Input: part model. Units: mm. Frame: model coordinates. A direction names the side the tool comes from. Give positions to 0.01 mm unless a question says otherwise; leave off trailing zeros. Loops run counter-clockwise (first coordinate to the right, second up) from the corner with the lowest first, then second, coordinate; pieces in that order, holes last. Notation, with made-up numbers: (-27, 37) -> (-18, 37) arc R5 ccw to (-18, 41) -> close; hole circle Ø8 at (-29, 60.25). An arc over 180 degrees is marked (long way). Answer as a JSON object with one key per item and string values. Group by question number.
```python
from build123d import *

# Parameters (mm, degrees)
SKETCH1_R                   = 11
FLANGE_DEPTH                = 2
SKETCH2_R                   = 5
COLLAR_DEPTH                = 10
SKETCH3_R                   = 3
CUT_EXTRUDE1_DEPTH          = 20.646882704
SET_SCREW_TAP_1_D           = 2.5
SET_SCREW_TAP_1_DEPTH       = 5
SET_SCREW_TAP_1_CSINK_D     = 2.55
SET_SCREW_TAP_1_CSINK_ANGLE = 90
SET_SCREW_TAP_2_D           = 2.5
SET_SCREW_TAP_2_DEPTH       = 8.001
SET_SCREW_TAP_2_CSINK_D     = 2.55
SET_SCREW_TAP_2_CSINK_ANGLE = 90
FLANGE_HOLES_AT_2_COUNT     = 2
FLANGE_HOLES_AT_2_PITCH     = 8
FLANGE_HOLES_AT_3_COUNT     = 2
FLANGE_HOLES_AT_3_PITCH     = 8
FLANGE_HOLES_AT_4_COUNT     = 2
FLANGE_HOLES_AT_4_PITCH     = 8
FLANGE_HOLES_AT_5_COUNT     = 2
FLANGE_HOLES_AT_5_PITCH     = 8
BODY_CHAMFERS_SIZE          = 0.2


with BuildPart() as part:
    # Sketch1 → Flange (new body)
    with BuildSketch(Plane(origin=(0, 0, 0), x_dir=(1, 0, 0), z_dir=(0, 1, 0))):
        with Locations(Location((0, 0, 0), (0, 0, 270))):
            Circle(SKETCH1_R)
    extrude(amount=FLANGE_DEPTH)

    # Sketch2 → Collar (add)
    with BuildSketch(Plane(origin=(0, 2, 0), x_dir=(1, 0, 0), z_dir=(0, 1, 0))):
        with Locations(Location((0, 0, 0), (0, 0, 270))):
            Circle(SKETCH2_R)
    extrude(amount=COLLAR_DEPTH)

    # Sketch3 → Cut-Extrude1 (cut, through all)
    with BuildSketch(Plane(origin=(0, 12, 0), x_dir=(1, 0, 0), z_dir=(0, 1, 0))):
        with Locations(Location((0, 0, 0), (0, 0, 270))):
            Circle(SKETCH3_R)
    extrude(amount=-CUT_EXTRUDE1_DEPTH, mode=Mode.SUBTRACT)

    # Set Screw Tap 1
    with Locations(Plane(origin=(5, 8.85, 0), x_dir=(0, 0, 1), z_dir=(1, 0, 0))):
        with Locations((0, 0)):
            CounterSinkHole(SET_SCREW_TAP_1_D / 2, SET_SCREW_TAP_1_CSINK_D / 2, depth=SET_SCREW_TAP_1_DEPTH, counter_sink_angle=SET_SCREW_TAP_1_CSINK_ANGLE)

    # Set Screw Tap 2
    with Locations(Plane(origin=(-5, 8.85, 0), x_dir=(0, 0, -1), z_dir=(-1, 0, 0))):
        with Locations((0, 0)):
            CounterSinkHole(SET_SCREW_TAP_2_D / 2, SET_SCREW_TAP_2_CSINK_D / 2, depth=SET_SCREW_TAP_2_DEPTH, counter_sink_angle=SET_SCREW_TAP_2_CSINK_ANGLE)

    # Sketch11 → Flange Holes (revolve, cut)
    with BuildSketch(Plane(origin=(0, 2, 0), x_dir=(0, 0, 1), z_dir=(1, 0, 0))):
        Polygon((0, 0), (0, 2), (1.625, 2), (1.5, 1.875), (1.5, 0.125), (1.625, 0), align=None)
    flange_holes = revolve(axis=Axis((0, 8.35, 0), (0, -1, 0)), mode=Mode.SUBTRACT)

    # Flange Holes at 2: Flange Holes ×2
    with Locations(*[Vector(-0.7071067811865476, 0, -0.7071067811865476) * (i * FLANGE_HOLES_AT_2_PITCH) for i in range(1, FLANGE_HOLES_AT_2_COUNT)]):
        add(flange_holes, mode=Mode.SUBTRACT)

    # Flange Holes at 3: Flange Holes ×2
    with Locations(*[Vector(-0.7071067811865476, 0, 0.7071067811865476) * (i * FLANGE_HOLES_AT_3_PITCH) for i in range(1, FLANGE_HOLES_AT_3_COUNT)]):
        add(flange_holes, mode=Mode.SUBTRACT)

    # Flange Holes at 4: Flange Holes ×2
    with Locations(*[Vector(0.7071067811865476, 0, 0.7071067811865476) * (i * FLANGE_HOLES_AT_4_PITCH) for i in range(1, FLANGE_HOLES_AT_4_COUNT)]):
        add(flange_holes, mode=Mode.SUBTRACT)

    # Flange Holes at 5: Flange Holes ×2
    with Locations(*[Vector(0.7071067811865476, 0, -0.7071067811865476) * (i * FLANGE_HOLES_AT_5_PITCH) for i in range(1, FLANGE_HOLES_AT_5_COUNT)]):
        add(flange_holes, mode=Mode.SUBTRACT)

    # Body Chamfers
    body_chamfers_edges = [part.edges().sort_by_distance(p)[0] for p in [
        (0, 0, -3),
        (0, 12, -3),
        (0, 0, -11),
        (0, 2, -11),
        (0, 2, -5),
        (0, 12, -5),
    ]]
    chamfer(body_chamfers_edges, length=BODY_CHAMFERS_SIZE)


solid = part.part
```
Q1. Set-up query: faces 5 (the face through (4.64, 1.01, -6.76)), 6 (the face through (3, 2, 5)). Return all of +Z, -Z, +X, -X, +Y, -Y with unobstructed straight access to the full face (end or side cutting, diameter ignored); none if empty.
Q2. Section D-D on y = 5.5. Return the cut outline in (x, z), then the cut area to 3 significant figures.
Q3. Section A-A on x = 0. Return the cut outline in (y, z).
Q4. Ray query, probe 1 along Y at (x, z) = (3.45, 0); probe 2 along Y at (x, z) = (-1.5, 5.75); probe 3 along X at (y, z) = (10, -1.25). Return the intervals inside material, ascending.
Q5. Section C-C on y = 9.5. Return the cut outline in (x, z).
Q6. Section B-B on z = 0. State how many separate pieces and enclosed holes the cut face has, then the cut area to 3 significant figures.
Q7. Pin query (flat end, axial travel): pin 1 Ø1.5 at (x, z) = (-7, 1.5) entering from -Y; pin 2 Ø3 at (y, z) = (10, -2.5) entering from -X; pin 3 Ø6 at (y, z) = (10.5, 7.5) entering from -X; pin 4 Ø2 at (x, y) = (-3, 4.5) entering from -Z. Return the tip coordinate at first contact, or that it passes through.
Q8. Pull-direction query (X, two-part tool) for faces 1 (the face through (4.17, 1.01, 5.46)), 2 (the face through (3.835, 9.959, -0.577)), 3 (the face through (-4.436, 6.933, 2.307)), 4 (the face through (-4.744, 1.012, -6.847)); classes: +X half, -X half, draft (parallel to the pull), parting line (faces both ways), or undercut.
Numbers:
{
 "1": {"face 5": "+Y, -Y", "face 6": "+Y"},
 "2": {"outline": "circle Ø10 at (0, 0); hole circle Ø6 at (0, 0)", "area": "50.3 mm²"},
 "3": {"outline": "(0, -10.8) -> (0.2, -11) -> (1.8, -11) -> (2, -10.8) -> (2, -5.2) -> (2.2, -5) -> (11.8, -5) -> (12, -4.8) -> (12, -3.2) -> (11.8, -3) -> (0.2, -3) -> (0, -3.2) -> close; (0, 3.2) -> (0.2, 3) -> (11.8, 3) -> (12, 3.2) -> (12, 4.8) -> (11.8, 5) -> (2.2, 5) -> (2, 5.2) -> (2, 10.8) -> (1.8, 11) -> (0.2, 11) -> (0, 10.8) -> close"},
 "4": {"probe 1": "y = 0 to 7.6, 10.1 to 12", "probe 2": "y = 0 to 2", "probe 3": "x = -4.84 to -2.73, 2.73 to 4.84"},
 "5": {"outline": "(-4.88, -1.07) arc R5 ccw to (4.88, -1.07) -> (2.8, -1.07) arc R3 cw to (-2.8, -1.07) -> close; (-4.88, 1.07) -> (-2.8, 1.07) arc R3 cw to (2.8, 1.07) -> (4.88, 1.07) arc R5 ccw to start"},
 "6": {"separate pieces": "4", "enclosed holes": "0", "area": "61.8 mm²"},
 "7": {"pin 1": "stops at y = 0", "pin 2": "stops at x = -4.9", "pin 3": "stops at x = -2.18", "pin 4": "stops at z = -4.58"},
 "8": {"face 1": "undercut", "face 2": "draft", "face 3": "parting line", "face 4": "undercut"}
}
